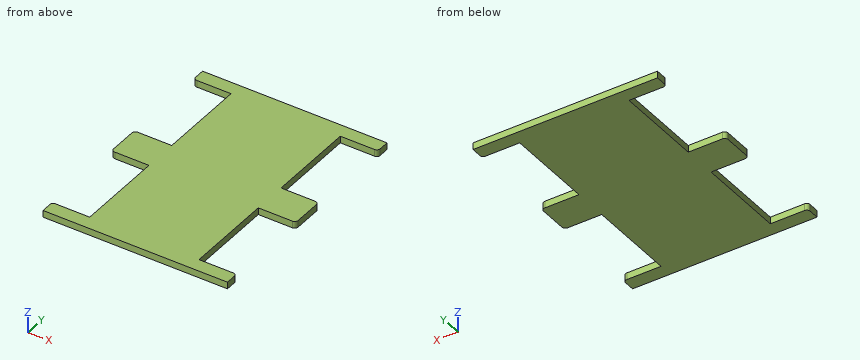
Solid Edge part; units mm, degrees
sketch "Sketch1" plane through (0, 0, 0) normal (0, -1, 0) x (1, 0, 0)
  line L0 (135, 0) -> (135, 10)
  line L1 (135, 10) -> (-135, 10)
  line L2 (-135, 10) -> (-135, 0)
  line L3 (-135, 0) -> (135, 0)
extrude "Protrusion1" add sketch "Sketch1" against normal blind 350
sketch "Sketch2" plane through (0, 175, 10) normal (0, 0, 1) x (1, 0, 0)
  line L0 (-135, 25) -> (-80, 25)
  line L1 (-80, 25) -> (-80, 155)
  line L2 (-80, 155) -> (-135, 155)
  line L3 (-135, 155) -> (-135, 25)
extrude "ExtrudedCutout_2" cut sketch "Sketch2" against normal blind 39.4331
mirror "Mirror1" about plane through (0, 0, 0) normal (1, 0, 0) of "ExtrudedCutout_2"
sketch "Sketch3" plane through (0, 175, 10) normal (0, 0, 1) x (1, 0, 0)
  line L0 (-135, -155) -> (-80, -155)
  line L1 (-80, -155) -> (-80, -25)
  line L2 (-80, -25) -> (-135, -25)
  line L3 (-135, -25) -> (-135, -155)
extrude "ExtrudedCutout_13" cut sketch "Sketch3" against normal blind 106.055
mirror "Mirror2" about plane through (0, 0, 0) normal (1, 0, 0) of "ExtrudedCutout_13"
fillet "Round_5" radius 5 4 edges at (135, 150, 5) (135, 200, 5) (-135, 150, 5) (-135, 200, 5)
fillet "Round_7" radius 5 4 edges at (135, 330, 5) (-135, 330, 5) (135, 20, 5) (-135, 20, 5)
Here's how the part is built. I have some questions about the finished solid (model axes, mm). Coordinates: 2 decimals unless noted, no trailing zeros. Order: outer loops, then holes, each group sorted by start corner. A loop starts at its lowest first (then second) coordinate and runs counter-clockwise, first axis right, second up.
Item 1: If we section it at A-A on x = 100: List the corners of the cut face in (y, z) for me, plus the area to 3 significant figures.
Result sheet:
outline: (0, 0) - (20, 0) - (20, 10) - (0, 10) - close; (150, 0) - (200, 0) - (200, 10) - (150, 10) - close; (330, 0) - (350, 0) - (350, 10) - (330, 10) - close
area: 900 mm2
Item 2: If we section it at C-C on y = 311: List the corners of the cut face in (x, z) for me, plus the area to 3 significant figures.
Result sheet:
outline: (-80, 0) - (80, 0) - (80, 10) - (-80, 10) - close
area: 1,600 mm2
Item 3: For P1, Ø3, axis at y = 85, z = 6, coming from the +X side; P2, Ø3, axis at y = 284.5, z = 7, coming from the -X side, each with a flat end and sliding along its axis, tell me the tip position at first contact or that it passes through.
Result sheet:
P1: stops at x = 80
P2: stops at x = -80
Item 4: I need wall thicknesses on line 1 (Y direction, x = -107, z = 3.25); line 2 (X direction, y = 66, z = 0.5). Which ranges of each line are inside material? Lowest first, please.
Result sheet:
line 1: y = 0 to 20, 150 to 200, 330 to 350
line 2: x = -80 to 80
Item 5: If we section it at B-B on z = 2.5: List the corners of the cut face in (x, y) for me, plus the area to 3 significant figures.
Result sheet:
outline: (-135, 0) - (135, 0) - (135, 15) arc R5 ccw to (130, 20) - (80, 20) - (80, 150) - (130, 150) arc R5 ccw to (135, 155) - (135, 195) arc R5 ccw to (130, 200) - (80, 200) - (80, 330) - (130, 330) arc R5 ccw to (135, 335) - (135, 350) - (-135, 350) - (-135, 335) arc R5 ccw to (-130, 330) - (-80, 330) - (-80, 200) - (-130, 200) arc R5 ccw to (-135, 195) - (-135, 155) arc R5 ccw to (-130, 150) - (-80, 150) - (-80, 20) - (-130, 20) arc R5 ccw to (-135, 15) - close
area: 65,900 mm2
